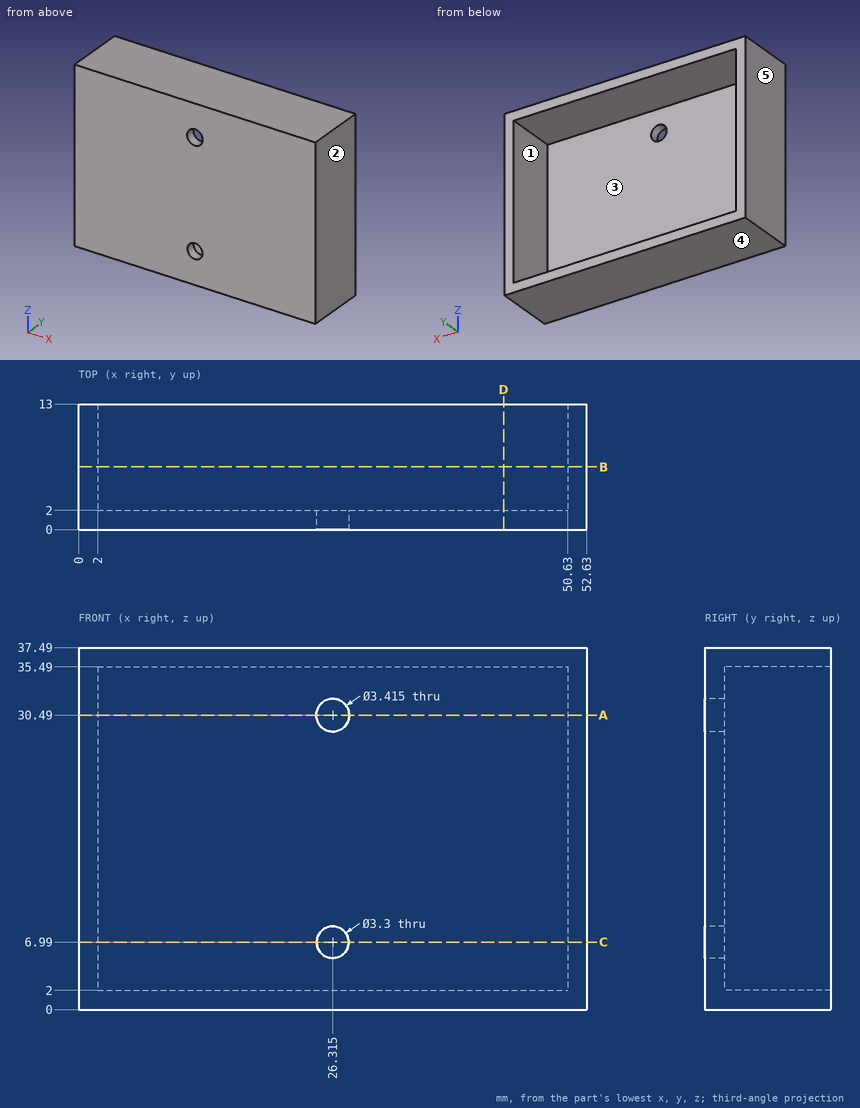
Verification items for this drawing (mm, ordinates from the low corner). A direction names the side the tool comes from. Coordinates: 2 decimals unless noted, no trailing zeros. Loops run counter-clockwise (first coordinate to the right, second up) from the corner with the lowest first, then second, coordinate; pieces in that order, holes last. Notation, with made-up numbers: (-32, 27) - (-20, 27) arc R29 ccw to (-20, 47) - close; hole circle Ø8 at (84.25, 62.25). An arc over 180 degrees is marked (long way). One line per item, written item: value. Start each with the question number.
(1) Depth check by flat-ended pin: P1, Ø16.5, axis at x = 34, z = 21, coming from the +Y side. Enter the tip coordinate at first touch or a pass-through.
(2) Cross-section at C-C on z = 6.99. Enter the section's corners in (x, y) (1 decimal), plus the area to 3 significant figures.
(3) Mould release check, pull along X, two halves, no side actions. Record for the marked faces 3, 4 and 5: released by +X, released by -X, zero draft, split by the parting line, or undercut.
(4) Cross-section at B-B on y = 6.5. Enter the section's corners in (x, z).
(5) Tool access check on the marked faces 1 and 2. Record the directions out of +Z, -Z, +X, -X, +Y, -Y that give a thin tool (end or side, any length) a straight path to the whole face; none if there is none.
(6) Material ranges on line 1 (X direction, y = 9, z = 7.5); line 2 (Z direction, x = 39, y = 7); line 3 (X direction, y = 0.75, z = 6.99) (1 decimal), recorded low to high. Write a range as [from, to].
(7) Cross-section at A-A on z = 30.49. Enter the section's corners in (x, y).
(8) Cross-section at D-D on x = 44. Enter the section's corners in (y, z).
Results below:
1. P1: stops at y = 2
2. outline: (0, 0) - (24.7, 0) - (24.7, 2) - (2, 2) - (2, 13) - (0, 13) - close; (28, 0) - (52.6, 0) - (52.6, 13) - (50.6, 13) - (50.6, 2) - (28, 2) - close
2. area: 143 mm2
3. face 3: undercut
3. face 4: zero draft
3. face 5: released by -X
4. outline: (0, 0) - (52.63, 0) - (52.63, 37.49) - (0, 37.49) - close; hole (2, 2) - (50.63, 2) - (50.63, 35.49) - (2, 35.49) - close
5. face 1: +Y
5. face 2: +Z, -Z, +X, +Y, -Y
6. line 1: x = [0, 2], [50.63, 52.63]
6. line 2: z = [0, 2], [35.49, 37.49]
6. line 3: x = [0, 24.7], [28, 52.6]
7. outline: (0, 0) - (24.61, 0) - (24.61, 2) - (2, 2) - (2, 13) - (0, 13) - close; (28.02, 0) - (52.63, 0) - (52.63, 13) - (50.63, 13) - (50.63, 2) - (28.02, 2) - close
8. outline: (0, 0) - (13, 0) - (13, 2) - (2, 2) - (2, 35.49) - (13, 35.49) - (13, 37.49) - (0, 37.49) - close
